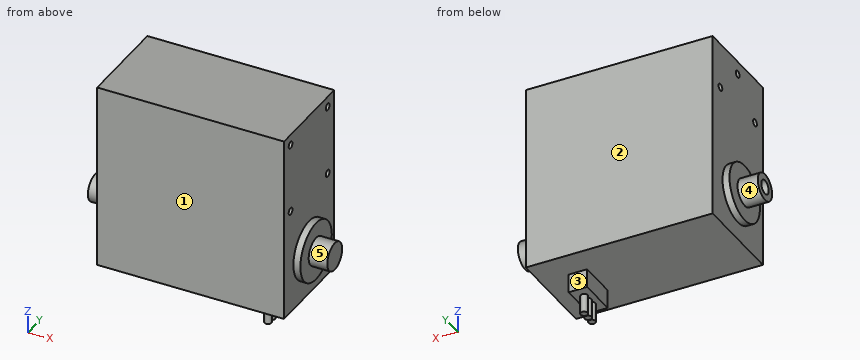
```python
from build123d import *

# Parameters (mm, degrees)
ESQUISSE1_W                       = 40.15
ESQUISSE1_H                       = 40.15
BOSS_EXTRU_1_DEPTH                = 10.15
ESQUISSE3_R                       = 6.15
BOSS_EXTRU_2_DEPTH                = 1.5
ESQUISSE4_R                       = 2.9
BOSS_EXTRU_3_DEPTH                = 4.35
DIAM_TRE_DU_PER_AGE_3_0_3_1_D     = 3
DIAM_TRE_DU_PER_AGE_3_0_3_1_DEPTH = 6
DIAM_TRE_DU_PER_AGE_3_0_3_1_TIP   = 0.901290929
ESQUISSE5_R                       = 6.35
BOSS_EXTRU_4_DEPTH                = 1.5
ESQUISSE6_R                       = 3
BOSS_EXTRU_5_DEPTH                = 4
ESQUISSE7_W                       = 4
ESQUISSE7_H                       = 8.3
BOSS_EXTRU_6_DEPTH                = 4
ESQUISSE8_R                       = 0.75
BOSS_EXTRU_8_DEPTH                = 4
ESQUISSE9_R                       = 0.75
ENL_V_MAT_EXTRU_1_DEPTH           = 5
ESQUISSE10_R                      = 0.75
ENL_V_MAT_EXTRU_2_DEPTH           = 5


with BuildPart() as part:
    # Esquisse1 → Boss.-Extru.1 (new, symmetric)
    with BuildSketch(Plane(origin=(0, 0, 0), x_dir=(1, 0, 0), z_dir=(0, 1, 0))):
        Rectangle(ESQUISSE1_W, ESQUISSE1_H)
    extrude(amount=BOSS_EXTRU_1_DEPTH, both=True)

    # Esquisse3 → Boss.-Extru.2 (add)
    with BuildSketch(Plane.ZY.offset(20.075)):
        with Locations(Location((-10.075, 0, 0), (0, 0, 180))):
            Circle(ESQUISSE3_R)
    extrude(amount=BOSS_EXTRU_2_DEPTH)

    # Esquisse4 → Boss.-Extru.3 (add)
    with BuildSketch(Plane.ZY.offset(21.575)):
        with Locations((-10.075, 0)):
            Circle(ESQUISSE4_R)
    extrude(amount=BOSS_EXTRU_3_DEPTH)

    # Diam_tre du per_age _3.0 _3_1
    with Locations(Plane.ZY.offset(25.925)):
        with Locations((-10.075, 0)):
            Hole(DIAM_TRE_DU_PER_AGE_3_0_3_1_D / 2, depth=DIAM_TRE_DU_PER_AGE_3_0_3_1_DEPTH)
            with Locations((0, 0, -(DIAM_TRE_DU_PER_AGE_3_0_3_1_DEPTH + DIAM_TRE_DU_PER_AGE_3_0_3_1_TIP / 2))):  # 118° drill point
                Cone(0, DIAM_TRE_DU_PER_AGE_3_0_3_1_D / 2, DIAM_TRE_DU_PER_AGE_3_0_3_1_TIP, mode=Mode.SUBTRACT)

    # Esquisse5 → Boss.-Extru.4 (add)
    with BuildSketch(Plane(origin=(20.075, 0, 0), x_dir=(0, 0, -1), z_dir=(1, 0, 0))):
        with Locations(Location((10.075, 0, 0), (0, 0, 180))):
            Circle(ESQUISSE5_R)
    extrude(amount=BOSS_EXTRU_4_DEPTH)

    # Esquisse6 → Boss.-Extru.5 (add)
    with BuildSketch(Plane(origin=(21.575, 0, 0), x_dir=(0, 0, -1), z_dir=(1, 0, 0))):
        with Locations((10.075, 0)):
            Circle(ESQUISSE6_R)
    extrude(amount=BOSS_EXTRU_5_DEPTH)

    # Esquisse7 → Boss.-Extru.6 (add)
    with BuildSketch(Plane(origin=(0, 0, -20.075), x_dir=(-1, 0, 0), z_dir=(0, 0, -1))):
        with Locations((-12.075, 0)):
            Rectangle(ESQUISSE7_W, ESQUISSE7_H)
    extrude(amount=BOSS_EXTRU_6_DEPTH)

    # Esquisse8 → Boss.-Extru.8 (add)
    with BuildSketch(Plane(origin=(0, 0, -24.075), x_dir=(-1, 0, 0), z_dir=(0, 0, -1))):
        with Locations((-12.075, 0)):
            Circle(ESQUISSE8_R)
        with Locations(Location((-12.075, -1.6, 0), (0, 0, 180))):
            Circle(ESQUISSE8_R)
        with Locations(Location((-12.075, 1.6, 0), (0, 0, 180))):
            Circle(ESQUISSE8_R)
    extrude(amount=BOSS_EXTRU_8_DEPTH)

    # Esquisse9 → Enl_v. mat.-Extru.1 (cut)
    with BuildSketch(Plane(origin=(20.075, 0, 0), x_dir=(0, 0, -1), z_dir=(1, 0, 0))):
        with Locations((-17.775, 7.5)):
            Circle(ESQUISSE9_R)
        with Locations((-2.775, 7.5)):
            Circle(ESQUISSE9_R)
        with Locations((-17.775, -7.5)):
            Circle(ESQUISSE9_R)
        with Locations((-2.775, -7.5)):
            Circle(ESQUISSE9_R)
    extrude(amount=-ENL_V_MAT_EXTRU_1_DEPTH, mode=Mode.SUBTRACT)

    # Esquisse10 → Enl_v. mat.-Extru.2 (cut)
    with BuildSketch(Plane.ZY.offset(20.075)):
        with Locations((17.275, 0)):
            Circle(ESQUISSE10_R)
        with Locations((10.275, 7)):
            Circle(ESQUISSE10_R)
        with Locations(Location((10.275, -7, 0), (0, 0, 180))):
            Circle(ESQUISSE10_R)
    extrude(amount=-ENL_V_MAT_EXTRU_2_DEPTH, mode=Mode.SUBTRACT)


solid = part.part
```
Could you check a few things on this model? Use its own coordinates, in mm. Face numbers are marked on the shaded views. A direction names the side the tool comes from. Round coordinates to 2 decimals unless told otherwise and drop trailing zeros. Write each loop counter-clockwise with the first axis right and the second up, starting at its lowest first coordinate (ties: lowest second). Pieces come first, ordered by that corner, then holes. Notation, with made-up numbers: M 2,-8 L 16,-8 A38 ccw 16,31 Z; hole C 89.25,48 d5. An arc over 180 degrees is marked long. Answer in a Markdown table with one row per item. Add a question column.
Q1. If I drill on line 1 (Z direction, x = -10.5, y = 1.5) (3 decimals); line 2 (X direction, y = 1.75, z = -6) (3 decimals), over which ranges is the centre line in solid material (lowest first)? Write a range as from..to.
Q2. Imagine slicing it at A-A (x = 18). Please give me the cut outline in (y, z) (3 decimals), then the cut area to 3 significant figures.
Q3. On a 3-axis mill with a long thin cutter (end or side, diameter ignored), from which of +Z, -Z, +X, -X, +Y, -Y can I reach the whole of each face in a straight line? I mean the marked faces 1, 2, 3, 4 and 5. Say none if no direction works.
Q4. Imagine slicing it at D-D (z = -14.5). Please give me the cut outline in (x, y) (3 decimals).
Q5. Will these pins go through, and if not, where does the flat tip stop? pin 1 Ø1.6 at (y, z) = (0, 17) entering from -X (3 decimals); pin 2 Ø6 at (x, y) = (2.5, -2) entering from -Z (3 decimals); pin 3 Ø2.5 at (y, z) = (7.5, 2.775) entering from +X (3 decimals).
Q6. Imagine slicing it at B-B (z = -5). Please give me the cut outline in (x, y) (3 decimals), then the cut area to 3 significant figures.
Q7. Imagine slicing it at C-C (x = 2). Please give me the cut outline in (y, z) (3 decimals), then the cut area to 3 significant figures.
Values:
| question | item | result |
|---|---|---|
| 1 | line 1 | -20.075..20.075 |
| 1 | line 2 | -21.575..21.575 |
| 2 | outline | M -10.15,-20.075 L 10.15,-20.075 L 10.15,20.075 L -10.15,20.075 Z; hole C -7.5,2.775 d1.5; hole C -7.5,17.775 d1.5; hole C 7.5,2.775 d1.5; hole C 7.5,17.775 d1.5 |
| 2 | area | 808 mm^2 |
| 3 | face 1 | +Z, -Z, +X, -X, -Y |
| 3 | face 2 | +Z, -Z, +X, -X, +Y |
| 3 | face 3 | -Z, +X, -X, +Y |
| 3 | face 4 | -X |
| 3 | face 5 | +X |
| 4 | outline | M -21.575,-4.271 L -20.075,-4.271 L -20.075,-10.15 L 20.075,-10.15 L 20.075,-4.554 L 21.575,-4.554 L 21.575,4.554 L 20.075,4.554 L 20.075,10.15 L -20.075,10.15 L -20.075,4.271 L -21.575,4.271 Z |
| 5 | pin 1 | x = -20.075 |
| 5 | pin 2 | z = -20.075 |
| 5 | pin 3 | x = 20.075 |
| 6 | outline | M -21.575,-3.474 L -20.075,-3.474 L -20.075,-10.15 L 20.075,-10.15 L 20.075,-3.817 L 21.575,-3.817 L 21.575,3.817 L 20.075,3.817 L 20.075,10.15 L -20.075,10.15 L -20.075,3.474 L -21.575,3.474 Z |
| 6 | area | 837 mm^2 |
| 7 | outline | M -10.15,-20.075 L 10.15,-20.075 L 10.15,20.075 L -10.15,20.075 Z |
| 7 | area | 815 mm^2 |
